Source: CAD feature listing. Evaluate the final solid. Frame: model axes, mm. A direction names the side the tool comes from. Round coordinates to 2 decimals unless told otherwise and drop trailing zeros. Loops run counter-clockwise (first coordinate to the right, second up) from the corner with the lowest first, then second, coordinate; pieces in that order, holes last.
Item 1: Access query for faces 4 (the flat face through (62, -10, -2)), 5 (the cylindrical face through (-14.985, 0.66, -39.44)), 6 (the flat face through (6, -14, 0)), 7 (the cylindrical face through (9.139, 14.334, -2.958)), 8 (the flat face through (13, -8, -80)). Directions: +Z, -Z, +X, -X, +Y, -Y. A direction counts if a zero-diameter tool reaches every point of the face in a straight line with its end or side. Return the directions, or none.
Item 2: Ray query, L1, parallel to Y at x = 80, z = 8.5; L2, parallel to Y at x = 0, z = -103; L3, parallel to X at y = 4, z = 2.5. Return the intervals inside material, ascending.
Item 3: Section query B-B on y = 10.5. Give the number of separate pieces and of enclosed holes in the cut face, then the cut area to 3 significant figures.
Item 4: Pull-direction query (X, two-part tool) for faces 1 (the cylindrical face through (60.02, 0.88, 16.79)), 2 (the cylindrical face through (51.93, -4.205, -55.438)), 3 (the flat face through (62, -10, 2)); classes: released by +X, released by -X, zero draft, split by the parting line, or undercut.
Item 5: Section query D-D on y = -23. Return loops of the section in (x, z), then the cut area to 3 significant figures.
Item 6: Section query A-A on x = -2. Return loops of the section in (y, z), then the cut area to 3 significant figures.
Item 7: First-contact query: P1, Ø8, axis at x = 49.5, y = 8, coming from the -Z side; P2, Ø12, axis at x = 86, z = 0.5, coming from the -Y side; P3, Ø8, axis at y = 12.5, z = -66, coming from the -X side. Flat tips, straight axial feed; report the tip coordinate or a pass-through.
```python
from build123d import *

# Parameters (mm, degrees)
F1_R      = 20
F4_R      = 17.55
F5_DEPTH  = 30
F6_R      = 15
F7_DEPTH  = 110.001
F8_R      = 20
F8_R_2    = 17
F9_DEPTH  = 6
F10_R     = 14
F12_R     = 27
F12_R_2   = 20
F13_DEPTH = 2
F14_DEPTH = 32
F15_R     = 14
F16_DEPTH = 34


with BuildPart() as f2:
    # F2: sweep along a path in F0
    with BuildLine(Plane.XZ) as f2_path:
        Line((0, 0), (0, -70))
        Line((0, -70), (0, -110))
    # F1 (on Top) → F2 (sweep)
    with BuildSketch(Plane.XY):
        Circle(F1_R)
    sweep(path=f2_path.line)

    # F3: sweep along a path in F0
    with BuildLine(Plane.XZ) as f3_path:
        Line((80, 0), (80, -23.8119784648))
        Line((80, -23.8119784648), (0, -70))
    # F1 (on Top) → F3 (sweep)
    with BuildSketch(Plane.XY):
        with Locations((80, 0)):
            Circle(F1_R)
    sweep(path=f3_path.line, transition=Transition.RIGHT)

    # F4 (on face) → F5 (cut)
    with BuildSketch(Plane(origin=(0, 0, -110), x_dir=(1, 0, 0), z_dir=(0, 0, -1))):
        Circle(F4_R)
    extrude(amount=-F5_DEPTH, mode=Mode.SUBTRACT)

    # F6 (on face) → F7 (cut, through all)
    with BuildSketch(Plane.XY):
        Circle(F6_R)
    extrude(amount=-F7_DEPTH, mode=Mode.SUBTRACT)

    # F8 (on face) → F9 (cut)
    with BuildSketch(Plane.XY):
        Circle(F8_R)
        Circle(F8_R_2, mode=Mode.SUBTRACT)
    extrude(amount=-F9_DEPTH, mode=Mode.SUBTRACT)

    # F11: sweep along a path in F0
    with BuildLine(Plane.XZ) as f11_path:
        Line((80, 0), (80, -23.8119784648))
        Line((80, -23.8119784648), (0, -70))
    # F10 (on face) → F11 (sweep, cut)
    with BuildSketch(Plane.XY):
        with Locations((80, 0)):
            Circle(F10_R)
    sweep(path=f11_path.line, transition=Transition.RIGHT, mode=Mode.SUBTRACT)

    # F12 (on face) → F13 (join, symmetric)
    with BuildSketch(Plane.XY):
        with Locations((80, 0)):
            Circle(F12_R)
        with Locations((80, 0)):
            Circle(F12_R_2, mode=Mode.SUBTRACT)
    extrude(amount=F13_DEPTH, both=True)

    # F1 (on Top) → F14 (join)
    with BuildSketch(Plane.XY):
        with Locations((80, 0)):
            Circle(F1_R)
    extrude(amount=F14_DEPTH)

    # F15 (on face) → F16 (cut)
    with BuildSketch(Plane.XY.offset(32)):
        with Locations((80, 0)):
            Circle(F15_R)
    extrude(amount=-F16_DEPTH, mode=Mode.SUBTRACT)


solid = f2.part
```
Data:
1. face 4: none
1. face 5: +Z, -Z
1. face 6: +Z, -X, +Y, -Y
1. face 7: +Z
1. face 8: -Z
2. L1: y = -20 to -14, 14 to 20
2. L2: y = -20 to -17.55, 17.55 to 20
2. L3: x = 60.4 to 66.58, 93.42 to 99.6
3. separate pieces: 3
3. enclosed holes: 0
3. area: 3,070 mm2
4. face 1: split by the parting line
4. face 2: undercut
4. face 3: zero draft
5. outline: (65.86, -2) - (94.14, -2) - (94.14, 2) - (65.86, 2) - close
5. area: 113 mm2
6. outline: (-19.9, -110) - (-17.44, -110) - (-17.44, -80) - (-14.87, -80) - (-14.87, 0) - (-16.88, 0) - (-16.88, -6) - (-19.9, -6) - close; (14.87, -80) - (17.44, -80) - (17.44, -110) - (19.9, -110) - (19.9, -6) - (16.88, -6) - (16.88, 0) - (14.87, 0) - close
6. area: 917 mm2
7. P1: stops at z = -65.45
7. P2: stops at y = -27
7. P3: stops at x = -18.1
